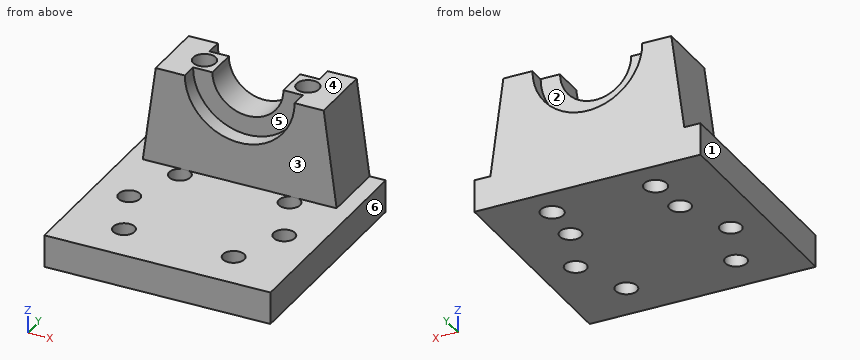
```python
from build123d import *

# Parameters (mm, degrees)
ESBO_O1_W                  = 50
ESBO_O1_H                  = 50
ESBO_O1_R                  = 1.65
RESSALTO_EXTRUS_O1_DEPTH   = 5
RESSALTO_EXTRUS_O2_START   = 15
RESSALTO_EXTRUS_O2_DEPTH   = 5
ESBO_O4_W                  = 8.5
ESBO_O4_H                  = 2.5
CORTE_EXTRUS_O1_DEPTH      = 39.405728739
CORTE_EXTRUS_O1_DEPTH_BACK = 39.405728739
ESBO_O5_W                  = 50
ESBO_O5_H                  = 50
ESBO_O5_W_2                = 35
ESBO_O5_H_2                = 35
ESBO_O6_R                  = 1.75
CORTE_EXTRUS_O2_DEPTH      = 34.260336739


with BuildPart() as part:
    # Esboço1 → Ressalto-extrusão1 (new body)
    with BuildSketch(Plane.XY):
        Rectangle(ESBO_O1_W, ESBO_O1_H)
        with Locations((12, 0)):
            Circle(ESBO_O1_R, mode=Mode.SUBTRACT)
        with Locations((8.485281374, -8.485281374)):
            Circle(ESBO_O1_R, mode=Mode.SUBTRACT)
        with Locations((-8.485281374, -8.485281374)):
            Circle(ESBO_O1_R, mode=Mode.SUBTRACT)
        with Locations((-12, 0)):
            Circle(ESBO_O1_R, mode=Mode.SUBTRACT)
        with Locations((-8.485281374, 8.485281374)):
            Circle(ESBO_O1_R, mode=Mode.SUBTRACT)
        with Locations((8.485281374, 8.485281374)):
            Circle(ESBO_O1_R, mode=Mode.SUBTRACT)
    extrude(amount=RESSALTO_EXTRUS_O1_DEPTH)

    # Esboço2 → Ressalto-extrusão2 (add, symmetric)
    with BuildSketch(Plane(origin=(0, 0, 0), x_dir=(1, 0, 0), z_dir=(0, 1, 0)).offset(RESSALTO_EXTRUS_O2_START)):
        with BuildLine():
            Line((13, -20), (15, -5))
            Line((15, -5), (-15, -5))
            Line((-15, -5), (-13, -20))
            Line((-13, -20), (-5.5, -20))
            ThreePointArc((-5.5, -20), (0, -14.5), (5.5, -20))
            Line((5.5, -20), (13, -20))
        make_face()
    extrude(amount=RESSALTO_EXTRUS_O2_DEPTH, both=True)

    # Esboço4 → Corte-Revolução3 (revolve, cut)
    with BuildSketch(Plane(origin=(0, 0, 0), x_dir=(0, 0, -1), z_dir=(1, 0, 0))):
        with Locations((-15.75, 18.75)):
            Rectangle(ESBO_O4_W, ESBO_O4_H)
        with Locations((-15.75, 11.25)):
            Rectangle(ESBO_O4_W, ESBO_O4_H)
    revolve(axis=Axis((0, 20, 20), (0, -1, 0)), mode=Mode.SUBTRACT)

    # Esboço5 → Corte-extrusão1 (cut, two sides: drawn at the far end of the back side and taken through both)
    with BuildSketch(Plane.XY.offset(5).offset(-CORTE_EXTRUS_O1_DEPTH_BACK)):
        Rectangle(ESBO_O5_W, ESBO_O5_H)
        with Locations((0, 2.5)):
            Rectangle(ESBO_O5_W_2, ESBO_O5_H_2, mode=Mode.SUBTRACT)
    extrude(amount=CORTE_EXTRUS_O1_DEPTH + CORTE_EXTRUS_O1_DEPTH_BACK, mode=Mode.SUBTRACT)

    # Esboço6 → Corte-extrusão2 (cut, through all)
    with BuildSketch(Plane.XY.offset(20)):
        with Locations((-8, 15)):
            Circle(ESBO_O6_R)
        with Locations((8, 15)):
            Circle(ESBO_O6_R)
    extrude(amount=-CORTE_EXTRUS_O2_DEPTH, mode=Mode.SUBTRACT)


solid = part.part
```
The model under review builds one solid part; all positions refer to its coordinate system, in mm. Face numbers are marked on the shaded views. A direction names the side the tool comes from. Round coordinates to 2 decimals unless told otherwise and drop trailing zeros. Write each loop counter-clockwise with the first axis right and the second up, starting at its lowest first coordinate (ties: lowest second). Pieces come first, ordered by that corner, then holes. Notation, with made-up numbers: (89, 32.5) - (131, 32.5) arc R31 ccw to (131, 63.5) - close; hole circle Ø10 at (-24, 60.5). An arc over 180 degrees is marked (long way). Answer as CSV lines item,"result". Start each with the question number.
(1) For pin 1 Ø4 at (x, z) = (12.5, 10) entering from -Y; pin 2 Ø3 at (x, y) = (10, -7) entering from -Z; pin 3 Ø2.5 at (x, z) = (2, 15) entering from -Y; pin 4 Ø6 at (x, y) = (-2, -10.5) entering from +Z, all flat-tipped, find the tip position at first contact; note any pin that passes through.
(2) We need section D-D on z = 11. State the section outline as (x, y) points, plus the area to 3 significant figures.
(3) To check wall thickness, follow line 1 (Y direction, x = 8, z = 12.25); line 2 (Y direction, x = -12, z = 1.8); line 3 (X direction, y = -0.5, z = 2.5). State the ranges of each line that lie inside material, in increasing order.
(4) For the marked faces 1, 2 and 3, list the 3-axis set-ups (+Z, -Z, +X, -X, +Y, -Y) from which the entire face can be reached by the end or side of a thin tool; tool diameter is ignored.
(5) We need section B-B on y = 15. State the section outline as (x, z) points.
(6) Draft analysis for pull direction X (two halves, no side actions). For the marked faces 4, 5 and 6, state which applies: pulls with the +X half, pulls with the -X half, needs draft (parallel to the pull), parting line crosses it, or undercut.
(7) We need section A-A on z = 17.25. State the section outline as (x, y) points, plus the area to 3 significant figures.
(8) We need section C-C on x = 12. State the section outline as (y, z) points.
Worked answers:
1,pin 1,"y = 10"
1,pin 2,"z = 0"
1,pin 3,"y = 12.5"
1,pin 4,"z = 5"
2,outline,"(-14.2, 10) - (14.2, 10) - (14.2, 20) - (-14.2, 20) - close; hole circle Ø3.5 at (-8, 15); hole circle Ø3.5 at (8, 15)"
2,area,"265 mm²"
3,line 1,"10 to 13.25, 16.75 to 20"
3,line 2,"-15 to -1.65, 1.65 to 20"
3,line 3,"-17.5 to -13.57, -10.43 to 10.43, 13.57 to 17.5"
4,face 1,"+Z, -Z, -X, +Y, -Y"
4,face 2,"+Z, +Y"
4,face 3,"+Z, +X, -X, -Y"
5,outline,"(-17.5, 0) - (-9.75, 0) - (-9.75, 20) - (-13, 20) - (-15, 5) - (-17.5, 5) - close; (-6.25, 0) - (6.25, 0) - (6.25, 20) - (5.5, 20) arc R5.5 cw to (-5.5, 20) - (-6.25, 20) - close; (9.75, 0) - (17.5, 0) - (17.5, 5) - (15, 5) - (13, 20) - (9.75, 20) - close"
6,face 4,"needs draft"
6,face 5,"undercut"
6,face 6,"pulls with the +X half"
7,outline,"(-13.37, 10) - (-8.04, 10) - (-8.04, 12.5) - (-4.76, 12.5) - (-4.76, 17.5) - (-8.04, 17.5) - (-8.04, 20) - (-13.37, 20) - close; (4.76, 12.5) - (8.04, 12.5) - (8.04, 10) - (13.37, 10) - (13.37, 20) - (8.04, 20) - (8.04, 17.5) - (4.76, 17.5) - close; hole circle Ø3.5 at (-8, 15); hole circle Ø3.5 at (8, 15)"
7,area,"120 mm²"
8,outline,"(-15, 0) - (-1.65, 0) - (-1.65, 5) - (-15, 5) - close; (1.65, 0) - (20, 0) - (20, 20) - (10, 20) - (10, 5) - (1.65, 5) - close"
